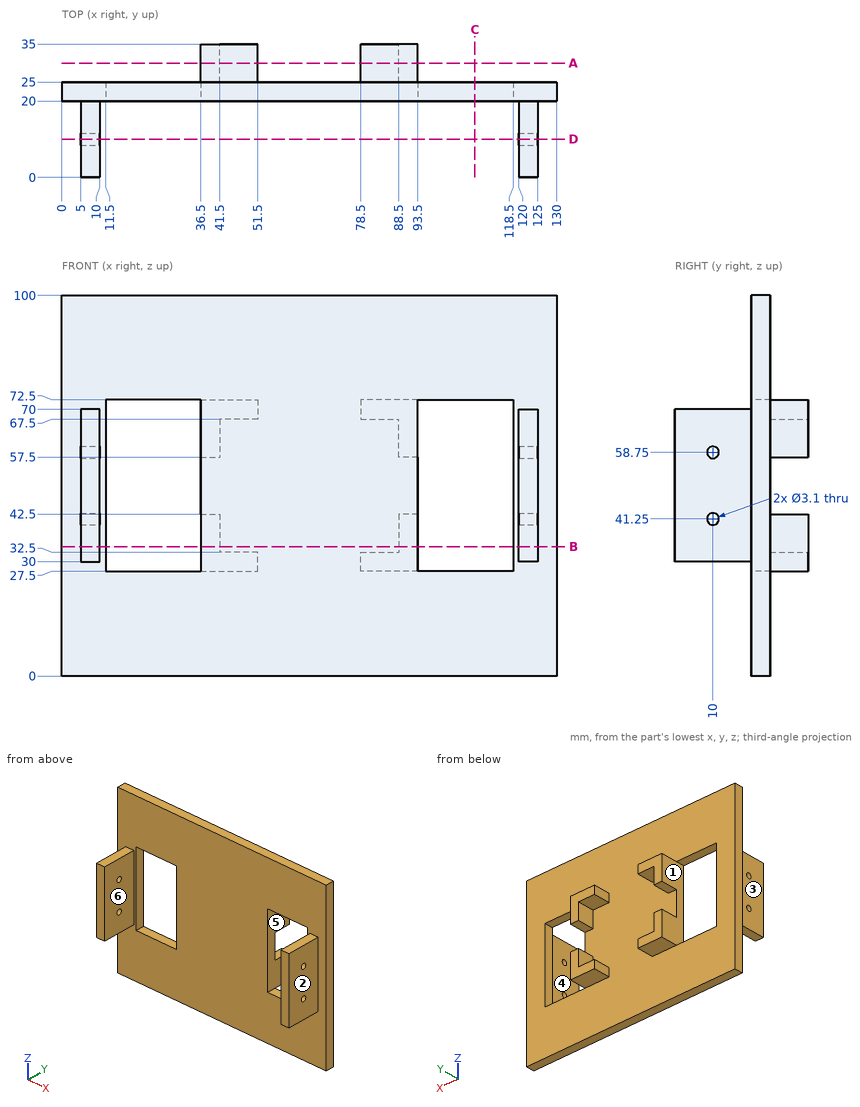
The figure shows three views and two pictorial views of one solid part (mm, origin at its lowest corner). Answer the questions. A direction names the side the tool comes from. Round coordinates to 2 decimals unless told otherwise and drop trailing zeros. Write each loop counter-clockwise with the first axis right and the second up, starting at its lowest first coordinate (ties: lowest second). Pieces come first, ordered by that corner, then holes. Notation, with made-up numbers: (-7.75, -29) -> (37.25, -29) arc R31 ccw to (37.25, -5) -> close; hole circle Ø3 at (37.5, 35.5). An arc over 180 degrees is marked (long way). Answer as a JSON object with one key per item and string values. Group by question number.
Q1. Section B-B (z = 34) is taken. Write down the section's boundary in (x, y).
Q2. Straight lines are drawn through the part: line 1 along Z through (x, y) = (123.5, 10); line 2 along X through (y, z) = (20.5, 49.5); line 3 along Y through (x, z) = (121, 41). For each, find the intervals that lie inside material, in ascending order.
Q3. Section C-C (x = 108.5) is taken. Write down the section's boundary in (y, z).
Q4. Determine the mould class of the marked faces 5 and 6 for opening direction Z: pulls with the +Z half, pulls with the -Z half, needs draft (parallel to the pull), parting line crosses it, or undercut.
Q5. Which of the six approach directions +Z, -Z, +X, -X, +Y, -Y give full straight-line access (tool end or side, diameter ignored) to the marked faces 1, 2, 3 and 4?
Q6. Section A-A (y = 30) is taken. Write down the section's boundary in (x, z).
Q7. Each of these flat-tipped pins is pushed along its axis until it touches: pin 1 Ø4 at (x, y) = (92, 31) entering from -Z; pin 2 Ø4 at (x, y) = (8.5, 12.5) entering from +Z; pin 3 Ø1.5 at (x, y) = (38.5, 31) entering from +Z. Where does it stop, or does it pass through?
Q8. Section D-D (y = 10) is taken. Write down the section's boundary in (x, z).
Check values:
{
 "1": {"outline": "(0, 20) -> (5, 20) -> (5, 0) -> (10, 0) -> (10, 20) -> (11.5, 20) -> (11.5, 25) -> (0, 25) -> close; (36.5, 20) -> (93.5, 20) -> (93.5, 35) -> (88.5, 35) -> (88.5, 25) -> (41.5, 25) -> (41.5, 35) -> (36.5, 35) -> close; (118.5, 20) -> (120, 20) -> (120, 0) -> (125, 0) -> (125, 20) -> (130, 20) -> (130, 25) -> (118.5, 25) -> close"},
 "2": {"line 1": "30 to 39.7, 42.8 to 57.2, 60.3 to 70", "line 2": "0 to 11.5, 36.5 to 93.5, 118.5 to 130", "line 3": "0 to 8.47, 11.53 to 25"},
 "3": {"outline": "(20, 0) -> (25, 0) -> (25, 27.5) -> (20, 27.5) -> close; (20, 72.5) -> (25, 72.5) -> (25, 100) -> (20, 100) -> close"},
 "4": {"face 5": "undercut", "face 6": "needs draft"},
 "5": {"face 1": "+Y, -Y", "face 2": "+Z, -Z, +X, -Y", "face 3": "+Z, -Z, -X, -Y", "face 4": "+Z, -Z, -Y"},
 "6": {"outline": "(36.5, 27.5) -> (51.5, 27.5) -> (51.5, 32.5) -> (41.5, 32.5) -> (41.5, 42.5) -> (36.5, 42.5) -> close; (36.5, 57.5) -> (41.5, 57.5) -> (41.5, 67.5) -> (51.5, 67.5) -> (51.5, 72.5) -> (36.5, 72.5) -> close; (78.5, 27.5) -> (93.5, 27.5) -> (93.5, 42.5) -> (88.5, 42.5) -> (88.5, 32.5) -> (78.5, 32.5) -> close; (78.5, 67.5) -> (88.5, 67.5) -> (88.5, 57.5) -> (93.5, 57.5) -> (93.5, 72.5) -> (78.5, 72.5) -> close"},
 "7": {"pin 1": "z = 27.5", "pin 2": "z = 70", "pin 3": "z = 72.5"},
 "8": {"outline": "(5, 30) -> (10, 30) -> (10, 39.7) -> (5, 39.7) -> close; (5, 42.8) -> (10, 42.8) -> (10, 57.2) -> (5, 57.2) -> close; (5, 60.3) -> (10, 60.3) -> (10, 70) -> (5, 70) -> close; (120, 30) -> (125, 30) -> (125, 39.7) -> (120, 39.7) -> close; (120, 42.8) -> (125, 42.8) -> (125, 57.2) -> (120, 57.2) -> close; (120, 60.3) -> (125, 60.3) -> (125, 70) -> (120, 70) -> close"}
}
